Design review of the part built by this model. Coordinates are the model's own, in mm. A direction names the side the tool comes from. Round coordinates to 2 decimals unless told otherwise and drop trailing zeros. Loops run counter-clockwise (first coordinate to the right, second up) from the corner with the lowest first, then second, coordinate; pieces in that order, holes last. Notation, with made-up numbers: (-39.5, -40) -> (-14.5, -40) arc R34 cw to (-14.5, -9) -> close; hole circle Ø9 at (75, 70). An arc over 180 degrees is marked (long way). Write each question's results on one line, items separated by ' | '. Start each with the question number.
from build123d import *

# Parameters (mm, degrees)
ESBO_O1_W                = 20
ESBO_O1_H                = 30
RESSALTO_EXTRUS_O1_DEPTH = 10
ESBO_O2_W                = 11
ESBO_O2_H                = 8
CORTE_EXTRUS_O1_DEPTH    = 10
ESBO_O3_W                = 11
ESBO_O3_H                = 6
CORTE_EXTRUS_O2_DEPTH    = 7
ESBO_O4_W                = 9
ESBO_O4_H                = 18
RESSALTO_EXTRUS_O2_DEPTH = 6.5
ESBO_O5_W                = 15.5
ESBO_O5_H                = 5.5
CORTE_EXTRUS_O3_DEPTH    = 7.5
ESBO_O6_R                = 2
CORTE_EXTRUS_O4_DEPTH    = 10
ESBO_O7_R                = 3.5
CORTE_EXTRUS_O5_DEPTH    = 2
FILETE1_R                = 6
FILETE2_R                = 3


with BuildPart() as part:
    # Esboço1 → Ressalto-extrusão1 (new body)
    with BuildSketch(Plane(origin=(0, 0, 0), x_dir=(1, 0, 0), z_dir=(0, 1, 0))):
        Rectangle(ESBO_O1_W, ESBO_O1_H)
    extrude(amount=RESSALTO_EXTRUS_O1_DEPTH)

    # Esboço2 → Corte-extrusão1 (cut)
    with BuildSketch(Plane(origin=(0, 10, 0), x_dir=(1, 0, 0), z_dir=(0, 1, 0))):
        with Locations((-4.5, 11)):
            Rectangle(ESBO_O2_W, ESBO_O2_H)
        with Locations((-4.5, -11)):
            Rectangle(ESBO_O2_W, ESBO_O2_H)
    extrude(amount=-CORTE_EXTRUS_O1_DEPTH, mode=Mode.SUBTRACT)

    # Esboço3 → Corte-extrusão2 (cut)
    with BuildSketch(Plane(origin=(0, 10, 0), x_dir=(1, 0, 0), z_dir=(0, 1, 0))):
        with Locations((-2, 0)):
            Rectangle(ESBO_O3_W, ESBO_O3_H)
    extrude(amount=-CORTE_EXTRUS_O2_DEPTH, mode=Mode.SUBTRACT)

    # Esboço4 → Ressalto-extrusão2 (add)
    with BuildSketch(Plane.XZ):
        with Locations((5.5, 0)):
            Rectangle(ESBO_O4_W, ESBO_O4_H)
    extrude(amount=RESSALTO_EXTRUS_O2_DEPTH)

    # Esboço5 → Corte-extrusão3 (cut)
    with BuildSketch(Plane(origin=(10, 0, 0), x_dir=(0, 0, -1), z_dir=(1, 0, 0))):
        with Locations((0, -2)):
            Rectangle(ESBO_O5_W, ESBO_O5_H)
    extrude(amount=-CORTE_EXTRUS_O3_DEPTH, mode=Mode.SUBTRACT)

    # Esboço6 → Corte-extrusão4 (cut, through all)
    with BuildSketch(Plane.ZY.offset(-1)):
        with Locations((11, 5)):
            Circle(ESBO_O6_R)
        with Locations((-11, 5)):
            Circle(ESBO_O6_R)
    extrude(amount=-CORTE_EXTRUS_O4_DEPTH, mode=Mode.SUBTRACT)

    # Esboço7 → Corte-extrusão5 (cut)
    with BuildSketch(Plane.ZY.offset(-1)):
        with Locations((11, 5)):
            Circle(ESBO_O7_R)
        with Locations((-11, 5)):
            Circle(ESBO_O7_R)
    extrude(amount=-CORTE_EXTRUS_O5_DEPTH, mode=Mode.SUBTRACT)

    # Filete1
    filete1_edges = [part.edges().sort_by_distance(p)[0] for p in [
        (-10, 5, -7),
        (-10, 5, 7),
    ]]
    fillet(filete1_edges, radius=FILETE1_R)

    # Filete2
    filete2_edges = [part.edges().sort_by_distance(p)[0] for p in [
        (5.5, 0, 15),
        (5.5, 10, 15),
        (5.5, 0, -15),
        (5.5, -6.5, -9),
        (5.5, -6.5, 9),
        (5.5, 10, -15),
    ]]
    fillet(filete2_edges, radius=FILETE2_R)


solid = part.part
1) To check wall thickness, follow line 1 (Y direction, x = 8, z = 5.25); line 2 (Z direction, x = 7.75, y = -0.5); line 3 (Z direction, x = -2, y = 9.25). State the ranges of each line that lie inside material, in increasing order. Write a range as from..to.
2) Take a section at B-B (y = 4). State how many separate pieces and enclosed holes the cut face has, plus the area to 3 significant figures.
3) Take a section at C-C (x = -3.5). Write out the cut boundary in (y, z), plus the area to 3 significant figures.
4) Take a section at D-D (y = -2.25). Write out the cut boundary in (x, z), plus the area to 4 significant figures.
5) The part is to be moulded in two halves that separate along X. For faces 4 (the face through (2.5, -2, 0)), 5 (the face through (3, 3, -9)), 6 (the face through (-2, 3, 0)), 7 (the face through (5.56, 9.14, -14.1)), say which applies: +X half, -X half, draft (parallel to the pull), parting line (faces both ways), or undercut.
6) Insertion check: pin 1 (3 mm diameter, centred on y = -3, z = -4, fed in from +X); pin 2 (4 mm diameter, centred on x = 7, y = 0, fed in from -Z); pin 3 (1.5 mm diameter, centred on y = -4.5, z = 5.5, fed in from -X). Each pin has a flat end and moves straight along its axis. Give the tip position at first contact, or say it passes through.
7) Take a section at A-A (z = -11). Write out the cut boundary in (x, y), plus the area to 3 significant figures.
8) For faces 1 (the face through (5, -2, 9)), 2 (the face through (5, 0, -11)), 3 (the face through (2, 2.9, -13.8)), list the 3-axis set-ups (+Z, -Z, +X, -X, +Y, -Y) from which the entire face can be reached by the end or side of a thin tool; tool diameter is ignored.
Geometry check:
1) line 1: y = -6.5..-4.75, 0.75..10 | line 2: z = -9..-7.75, 7.75..9 | line 3: z = -7..-3, 3..7
2) separate pieces: 3 | enclosed holes: 1 | area: 267 mm^2
3) outline: (0, -7) -> (10, -7) -> (10, -3) -> (3, -3) -> (3, 3) -> (10, 3) -> (10, 7) -> (0, 7) -> close | area: 98.0 mm^2
4) outline: (1, -9) -> (10, -9) -> (10, -7.75) -> (2.5, -7.75) -> (2.5, 7.75) -> (10, 7.75) -> (10, 9) -> (1, 9) -> close | area: 45.75 mm^2
5) face 4: +X half | face 5: -X half | face 6: undercut | face 7: draft
6) pin 1: stops at x = 2.5 | pin 2: stops at z = -14.83 | pin 3: stops at x = 1
7) outline: (1, 0) -> (10, 0) -> (10, 3) -> (3, 3) -> (3, 1.5) -> (1, 1.5) -> close; (1, 8.5) -> (3, 8.5) -> (3, 7) -> (10, 7) -> (10, 10) -> (1, 10) -> close | area: 48.0 mm^2
8) face 1: +Z, +X, -X, -Y | face 2: -Z, +X, -X, -Y | face 3: -X
